Verification items for the finished model (mm, model axes). Face numbers are marked on the shaded views. A direction names the side the tool comes from. Round coordinates to 2 decimals unless told otherwise and drop trailing zeros. Write each loop counter-clockwise with the first axis right and the second up, starting at its lowest first coordinate (ties: lowest second). Pieces come first, ordered by that corner, then holes. Notation, with made-up numbers: (-13.5, 0) - (5.5, 0) arc R26 ccw to (5.5, 15) - close; hole circle Ø8 at (-38.75, 75). An arc over 180 degrees is marked (long way). Answer as a JSON object with one key per item and string values.
```python
from build123d import *

# Parameters (mm, degrees)
F0_R          = 11.1
F1_DEPTH      = 7
F2_W          = 5
F2_H          = 30
F3_DEPTH      = 10
F4_R          = 1.7
F5_DEPTH      = 5.001
F6_R          = 3.25
F7_DEPTH      = 2.5
F8_R          = 1.7
F9_DEPTH      = 25.001
F10_R         = 3.25
F11_DEPTH     = 2.5
F12_R         = 7.5
F13_DEPTH     = 1.6
F14_R         = 1
F15_R         = 1.7
F16_DEPTH     = 7.001
F17_R         = 3.25
F18_DEPTH     = 3
F19_T1_DEPTH  = 6.5
F19_T3_DEPTH  = 6.5
F19_S7_W      = 1
F19_S7_H      = 1
F19_T8_DEPTH  = 1
F19_S13_W     = 1
F19_S13_H     = 1
F19_T14_DEPTH = 1
F19_S19_W     = 1
F19_S19_H     = 1
F19_T20_DEPTH = 1
F19_S25_W     = 1
F19_S25_H     = 1
F19_T26_DEPTH = 1


# Not quite as in the source:
# - a fillet or chamfer that OpenCascade refuses, or shapes differently, is made with other operations: its cross-section is extruded or revolved along the edge and cut away or added


with BuildPart() as f1:
    # F0 (on Top) → F1 (new body)
    with BuildSketch(Plane.XY):
        with BuildLine():
            Line((-47.15, -15), (0, -15))
            ThreePointArc((0, -15), (15, 0), (0, 15))
            Line((0, 15), (-47.15, 15))
            Line((-47.15, 15), (-47.15, -15))
        make_face()
        Circle(F0_R, mode=Mode.SUBTRACT)
    extrude(amount=F1_DEPTH)

    # F2 (on face) → F3 (join)
    with BuildSketch(Plane.XY.offset(7)):
        with Locations((-44.65, 0)):
            Rectangle(F2_W, F2_H)
        with Locations((-24.65, 0)):
            Rectangle(F2_W, F2_H)
    extrude(amount=F3_DEPTH)

    # F4 (on face) → F5 (cut, through all)
    with BuildSketch(Plane.YZ.offset(-42.15)):
        with Locations((7.5, 12)):
            Circle(F4_R)
        with Locations((-7.5, 12)):
            Circle(F4_R)
    extrude(amount=-F5_DEPTH, mode=Mode.SUBTRACT)

    # F6 (on face) → F7 (cut)
    with BuildSketch(Plane(origin=(-47.15, 0, 0), x_dir=(0, -1, 0), z_dir=(-1, 0, 0))):
        with Locations((-7.5, 12)):
            Circle(F6_R)
        with Locations((7.5, 12)):
            Circle(F6_R)
    extrude(amount=-F7_DEPTH, mode=Mode.SUBTRACT)

    # F8 (on face) → F9 (cut, through all)
    with BuildSketch(Plane.YZ.offset(-22.15)):
        with Locations((7.5, 12)):
            Circle(F8_R)
        with Locations((-7.5, 12)):
            Circle(F8_R)
    extrude(amount=-F9_DEPTH, mode=Mode.SUBTRACT)

    # F10 (on face) → F11 (cut)
    with BuildSketch(Plane.YZ.offset(-22.15)):
        with Locations((7.5, 12)):
            Circle(F10_R)
        with Locations((-7.5, 12)):
            Circle(F10_R)
    extrude(amount=-F11_DEPTH, mode=Mode.SUBTRACT)

    # F12 (on face) → F13 (join)
    with BuildSketch(Plane.XY.offset(7)):
        with BuildLine():
            ThreePointArc((0, -15), (15, 0), (0, 15))
            Line((0, 15), (-22.15, 15))
            Line((-22.15, 15), (-22.15, -15))
            Line((-22.15, -15), (0, -15))
        make_face()
        Circle(F12_R, mode=Mode.SUBTRACT)
    extrude(amount=F13_DEPTH)

    # F14
    f14_edges = [f1.edges().sort_by_distance(p)[0] for p in [
        (-47.15, 0, 0),
        (-23.575, -15, 0),
        (15, 0, 0),
        (-23.575, 15, 0),
        (-47.15, -15, 8.5),
        (-47.15, 15, 8.5),
        (-47.15, 0, 17),
        (-22.15, 0, 17),
        (-22.15, -15, 12.8),
        (-22.15, 15, 12.8),
    ]]
    fillet(f14_edges, radius=F14_R)

    # F15 (on face) → F16 (cut, through all)
    with BuildSketch(Plane.XY.offset(7)):
        with Locations((-34.65, -7.5)):
            Circle(F15_R)
        with Locations((-34.65, 7.5)):
            Circle(F15_R)
    extrude(amount=-F16_DEPTH, mode=Mode.SUBTRACT)

    # F17 (on face) → F18 (cut)
    with BuildSketch(Plane.XY.offset(7)):
        with Locations((-34.65, -7.5)):
            Circle(F17_R)
        with Locations((-34.65, 7.5)):
            Circle(F17_R)
    extrude(amount=-F18_DEPTH, mode=Mode.SUBTRACT)

    # F19: fillet of radius 1 on 4 edges, made by hand

    # F19_s2 → F19_t1 (cut)
    with BuildSketch(Plane.YZ.offset(-46.15)):
        with BuildLine():
            ThreePointArc((15, 16), (14.7071067812, 16.7071067812), (14, 17))
            Line((14, 17), (15, 17))
            Line((15, 17), (15, 16))
        make_face()
        with BuildLine():
            ThreePointArc((-14, 17), (-14.7071067812, 16.7071067812), (-15, 16))
            Line((-15, 16), (-15, 17))
            Line((-15, 17), (-14, 17))
        make_face()
    extrude(amount=F19_T1_DEPTH, mode=Mode.SUBTRACT)

    # F19_s4 → F19_t3 (cut)
    with BuildSketch(Plane.YZ.offset(-29.65)):
        with BuildLine():
            ThreePointArc((15, 16), (14.7071067812, 16.7071067812), (14, 17))
            Line((14, 17), (15, 17))
            Line((15, 17), (15, 16))
        make_face()
        with BuildLine():
            ThreePointArc((-14, 17), (-14.7071067812, 16.7071067812), (-15, 16))
            Line((-15, 16), (-15, 17))
            Line((-15, 17), (-14, 17))
        make_face()
    extrude(amount=F19_T3_DEPTH, mode=Mode.SUBTRACT)


with BuildPart() as f19_tool6:
    # F19_s7 → F19_t8 (new body)
    with BuildSketch(Plane.XY.offset(16)):
        with Locations((-46.65, -14.5)):
            Rectangle(F19_S7_W, F19_S7_H)
    extrude(amount=F19_T8_DEPTH)

    # F19_s9 → F19_t10 (revolve, cut)
    with BuildSketch(Plane(origin=(-46.15, -14, 16), x_dir=(0.7071067812, 0.7071067812, 0), z_dir=(0.7071067812, -0.7071067812, 0))):
        with BuildLine():
            ThreePointArc((0, -1), (1, 0), (0, 1))
            Line((0, 1), (0, -1))
        make_face()
    revolve(axis=Axis((-46.15, -14, 16), (0, 0, 1)), mode=Mode.SUBTRACT)


with BuildPart() as f1_1:
    add(f1.part)

    # F19_t5: cut F19_tool6
    add(f19_tool6.part, mode=Mode.SUBTRACT)


with BuildPart() as f19_tool12:
    # F19_s13 → F19_t14 (new body)
    with BuildSketch(Plane.XY.offset(16)):
        with Locations((-22.65, -14.5)):
            Rectangle(F19_S13_W, F19_S13_H)
    extrude(amount=F19_T14_DEPTH)

    # F19_s15 → F19_t16 (revolve, cut)
    with BuildSketch(Plane(origin=(-23.15, -14, 16), x_dir=(-0.7071067812, 0.7071067812, 0), z_dir=(0.7071067812, 0.7071067812, 0))):
        with BuildLine():
            ThreePointArc((0, -1), (1, 0), (0, 1))
            Line((0, 1), (0, -1))
        make_face()
    revolve(axis=Axis((-23.15, -14, 16), (0, 0, 1)), mode=Mode.SUBTRACT)


with BuildPart() as f1_2:
    add(f1_1.part)

    # F19_t11: cut F19_tool12
    add(f19_tool12.part, mode=Mode.SUBTRACT)


with BuildPart() as f19_tool18:
    # F19_s19 → F19_t20 (new body)
    with BuildSketch(Plane.XZ.offset(-14)):
        with Locations((-22.65, 16.5)):
            Rectangle(F19_S19_W, F19_S19_H)
    extrude(amount=-F19_T20_DEPTH)

    # F19_s21 → F19_t22 (revolve, cut)
    with BuildSketch(Plane(origin=(-23.15, 14, 16), x_dir=(-0.7071067812, 0, -0.7071067812), z_dir=(0.7071067812, 0, -0.7071067812))):
        with BuildLine():
            ThreePointArc((0, -1), (1, 0), (0, 1))
            Line((0, 1), (0, -1))
        make_face()
    revolve(axis=Axis((-23.15, 14, 16), (0, 1, 0)), mode=Mode.SUBTRACT)


with BuildPart() as f1_3:
    add(f1_2.part)

    # F19_t17: cut F19_tool18
    add(f19_tool18.part, mode=Mode.SUBTRACT)


with BuildPart() as f19_tool24:
    # F19_s25 → F19_t26 (new body)
    with BuildSketch(Plane.XZ.offset(-14)):
        with Locations((-46.65, 16.5)):
            Rectangle(F19_S25_W, F19_S25_H)
    extrude(amount=-F19_T26_DEPTH)

    # F19_s27 → F19_t28 (revolve, cut)
    with BuildSketch(Plane(origin=(-46.15, 14, 16), x_dir=(0.7071067812, 0, -0.7071067812), z_dir=(0.7071067812, 0, 0.7071067812))):
        with BuildLine():
            ThreePointArc((0, -1), (1, 0), (0, 1))
            Line((0, 1), (0, -1))
        make_face()
    revolve(axis=Axis((-46.15, 14, 16), (0, 1, 0)), mode=Mode.SUBTRACT)


with BuildPart() as f1_4:
    add(f1_3.part)

    # F19_t23: cut F19_tool24
    add(f19_tool24.part, mode=Mode.SUBTRACT)


solid = f1_4.part
```
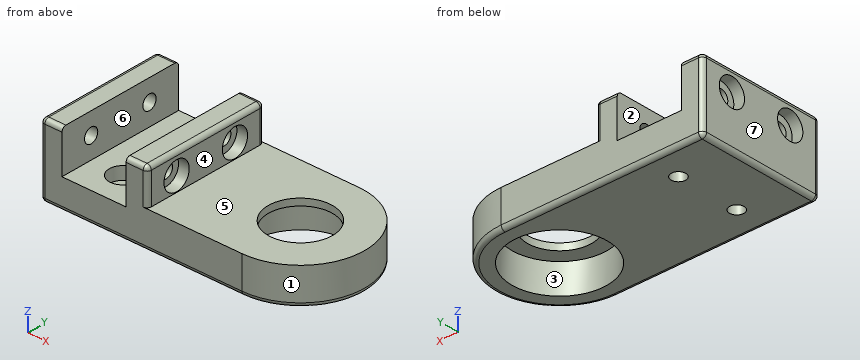
Q1. Section check A-A, the plane y = 0. Record the cut outline in (x, z), then the cut area to 3 significant figures.
Geometry check:
{"outline": "(-47.15, 1) arc R1 ccw to (-46.15, 0) - (-11.1, 0) - (-11.1, 7) - (-7.5, 7) - (-7.5, 8.6) - (-22.15, 8.6) - (-22.15, 16) arc R1 ccw to (-23.15, 17) - (-27.15, 17) - (-27.15, 7) - (-42.15, 7) - (-42.15, 17) - (-46.15, 17) arc R1 ccw to (-47.15, 16) - close; (7.5, 7) - (11.1, 7) - (11.1, 0) - (14, 0) arc R1 ccw to (15, 1) - (15, 8.6) - (7.5, 8.6) - close", "area": "414 mm2"}
Q2. Material ranges on line 1 along Y through (x, z) = (-34.65, 1.15); line 2 along Z through (x, y) = (-24, -7.5); line 3 along X through (y, z) = (1.75, 12.75), recorded low to high. Write a range as [from, to].
Geometry check:
{"line 1": "y = [-15, -9.2], [-5.8, 5.8], [9.2, 15]", "line 2": "z = [0, 8.75], [15.25, 17]", "line 3": "x = [-47.15, -42.15], [-27.15, -22.15]"}
Q3. Release check for a two-part mould opening along X. For the marked faces 5, 6 and 7 record: released by +X, released by -X, zero draft, split by the parting line, or undercut.
Geometry check:
{"face 5": "zero draft", "face 6": "undercut", "face 7": "released by -X"}
Q4. Section check B-B, the plane x = -43. Record the cut outline in (y, z).
Geometry check:
{"outline": "(-15, 1) arc R1 ccw to (-14, 0) - (14, 0) arc R1 ccw to (15, 1) - (15, 16) arc R1 ccw to (14, 17) - (-14, 17) arc R1 ccw to (-15, 16) - close; hole circle Ø3.4 at (-7.5, 12); hole circle Ø3.4 at (7.5, 12)"}
Q5. Section check C-C, the plane x = -5.5. Record the cut outline in (y, z), then the cut area to 3 significant figures.
Geometry check:
{"outline": "(-15, 1) arc R1 ccw to (-14, 0) - (-9.64, 0) - (-9.64, 7) - (-5.1, 7) - (-5.1, 8.6) - (-15, 8.6) - close; (5.1, 7) - (9.64, 7) - (9.64, 0) - (14, 0) arc R1 ccw to (15, 1) - (15, 8.6) - (5.1, 8.6) - close", "area": "106 mm2"}
Q6. Set-up check for the marked faces 1, 2, 3 and 4: record each of +Z, -Z, +X, -X, +Y, -Y from which the full face is reachable in a straight line by a thin tool's end or side.
Geometry check:
{"face 1": "+Z, -Z, +X", "face 2": "+Z, +Y, -Y", "face 3": "-Z", "face 4": "+Z, +X, +Y, -Y"}
Q7. Section check D-D, the plane z = 12. State how many separate pieces and enclosed holes the cut face has, then the cut area to 3 significant figures.
Geometry check:
{"separate pieces": "6", "enclosed holes": "0", "area": "200 mm2"}
Q8. Gauge pin test, flat ends, axial feed: P1, Ø4, axis at x = 5, y = -5, coming from the +Z side; P2, Ø3.5, axis at y = -6.5, z = 13.5, coming from the +X side; P3, Ø2, axis at y = -7.5, z = 12, coming from the +X side; P4, Ø17, axis at x = 0, y = 0, coming from the -Z side. Record the tip position at first contact, or that the pin passes through.
Geometry check:
{"P1": "stops at z = 8.6", "P2": "stops at x = -22.15", "P3": "passes through", "P4": "stops at z = 7"}
